Work out the finished part from the listing and answer in its coordinate system (mm). A direction names the side the tool comes from. Round coordinates to 2 decimals unless told otherwise and drop trailing zeros. Order: outer loops, then holes, each group sorted by start corner. A loop starts at its lowest first (then second) coordinate and runs counter-clockwise, first axis right, second up. Notation, with made-up numbers: (54.25, 12.25) - (105.25, 12.25) arc R28 ccw to (105.25, 39.25) - close; hole circle Ø9 at (74.25, -3.5). An arc over 180 degrees is marked (long way). Put each result on its own line as item: value.
```python
from build123d import *

# Parameters (mm, degrees)
SKETCH_1_W          = 55
SKETCH_1_H          = 100
EXTRUDE_1_DEPTH     = 30
CUT_EXTRUDE_1_DEPTH = 81.156097709
SKETCH_3_W          = 50
SKETCH_3_H          = 95
CUT_EXTRUDE_2_DEPTH = 25
FILLET_1_R          = 5
SKETCH_5_R          = 3
EXTRUDE_2_DEPTH     = 25
SKETCH_6_W          = 15
SKETCH_6_H          = 23
CUT_EXTRUDE_4_DEPTH = 5
CHAMFER_1_SIZE      = 4
SKETCH_7_R          = 5
EXTRUDE_3_DEPTH     = 5
SKETCH_8_R          = 2.75
CUT_EXTRUDE_5_DEPTH = 5


with BuildPart() as part:
    # 草圖1 → 填料-伸長1 (new body)
    with BuildSketch(Plane.XY):
        Rectangle(SKETCH_1_W, SKETCH_1_H)
    extrude(amount=EXTRUDE_1_DEPTH)

    # 草圖2 → 除料-伸長1 (cut, through all)
    with BuildSketch(Plane.ZY.offset(27.5)):
        with BuildLine():
            Line((13, 39.5), (30, 39.5))
            Line((30, 39.5), (30, 30.5))
            Line((30, 30.5), (13, 30.5))
            ThreePointArc((13, 30.5), (8.5, 35), (13, 39.5))
        make_face()
    extrude(amount=-CUT_EXTRUDE_1_DEPTH, mode=Mode.SUBTRACT)

    # 草圖3 → 除料-伸長2 (cut)
    with BuildSketch(Plane.XY.offset(30)):
        Rectangle(SKETCH_3_W, SKETCH_3_H)
    extrude(amount=-CUT_EXTRUDE_2_DEPTH, mode=Mode.SUBTRACT)

    # 圓角1
    fillet_1_edges = [part.edges().sort_by_distance(p)[0] for p in [
        (25, 47.5, 17.5),
        (-25, -47.5, 17.5),
        (25, -47.5, 17.5),
        (-25, 47.5, 17.5),
        (27.5, -50, 15),
        (-27.5, -50, 15),
        (-27.5, 50, 15),
        (27.5, 50, 15),
    ]]
    fillet(fillet_1_edges, radius=FILLET_1_R)

    # 草圖5 → 填料-伸長2 (add)
    with BuildSketch(Plane.XY.offset(5)):
        with Locations(Location((11, -35, 0), (0, 0, 180))):
            Circle(SKETCH_5_R)
    extrude(amount=EXTRUDE_2_DEPTH)

    # 草圖6 → 除料-伸長4 (cut)
    with BuildSketch(Plane.XZ.offset(50)):
        with Locations((0, 18.5)):
            Rectangle(SKETCH_6_W, SKETCH_6_H)
    extrude(amount=-CUT_EXTRUDE_4_DEPTH, mode=Mode.SUBTRACT)

    # 導角1
    # the kernel refuses this chamfer: 4 mm, written as the material it adds along each edge
    with BuildSketch(Plane(origin=(-20, -42.5, 5), x_dir=(-1, 0, 0), z_dir=(0, 1, 0))) as chamfer_1_piece_1:
        Polygon((5, CHAMFER_1_SIZE), (5 - CHAMFER_1_SIZE, 0), (5, 0), align=None)
    revolve(axis=Axis((-20, -42.5, 5), (0, 0, 1)), revolution_arc=90)
    with BuildSketch(Plane(origin=(-25, 42.5, 5), x_dir=(-0.027495876610586487, 0, 0.9996219169112968), z_dir=(0, -1, 0))) as chamfer_1_piece_2_section:
        Polygon((CHAMFER_1_SIZE * 0.999621916911, -CHAMFER_1_SIZE * 0.0274958766106), (-CHAMFER_1_SIZE * 0.0274958766106, -CHAMFER_1_SIZE * 0.999621916911), (0, 0), align=None)
    chamfer_1_piece_2 = extrude(amount=85, mode=Mode.PRIVATE)
    chamfer_1_piece_2 = chamfer_1_piece_2 - Plane(origin=(-23.679821879, 35, 13), x_dir=(0, -1, 0), z_dir=(-1, 0, 0)) * Cylinder(4.5, 186, mode=Mode.PRIVATE)
    add(chamfer_1_piece_2)
    with BuildSketch(Plane(origin=(-20, 42.5, 5), x_dir=(-1, 0, 0), z_dir=(0, -1, 0))) as chamfer_1_piece_3:
        Polygon((5 - CHAMFER_1_SIZE, 0), (5, -CHAMFER_1_SIZE), (5, 0), align=None)
    revolve(axis=Axis((-20, 42.5, 5), (0, 0, -1)), revolution_arc=90)
    with BuildSketch(Plane(origin=(20, 47.5, 5), x_dir=(0, -0.9996219169112968, -0.027495876610586296), z_dir=(-1, 0, 0))) as chamfer_1_piece_4:
        Polygon((CHAMFER_1_SIZE * 0.999621916911, CHAMFER_1_SIZE * 0.0274958766106), (-CHAMFER_1_SIZE * 0.0274958766106, CHAMFER_1_SIZE * 0.999621916911), (0, 0), align=None)
    extrude(amount=40)
    with BuildSketch(Plane(origin=(20, 42.5, 5), x_dir=(1, 0, 0), z_dir=(0, -1, 0))) as chamfer_1_piece_5:
        Polygon((5 - CHAMFER_1_SIZE, 0), (5, CHAMFER_1_SIZE), (5, 0), align=None)
    revolve(axis=Axis((20, 42.5, 5), (0, 0, 1)), revolution_arc=90)
    with BuildSketch(Plane(origin=(25, -42.5, 5), x_dir=(0.027495876610586487, 0, 0.9996219169112968), z_dir=(0, 1, 0))) as chamfer_1_piece_6_section:
        Polygon((CHAMFER_1_SIZE * 0.999621916911, -CHAMFER_1_SIZE * 0.0274958766106), (-CHAMFER_1_SIZE * 0.0274958766106, -CHAMFER_1_SIZE * 0.999621916911), (0, 0), align=None)
    chamfer_1_piece_6 = extrude(amount=85, mode=Mode.PRIVATE)
    chamfer_1_piece_6 = chamfer_1_piece_6 - Plane(origin=(23.679821879, 35, 13), x_dir=(0, -1, 0), z_dir=(-1, 0, 0)) * Cylinder(4.5, 186, mode=Mode.PRIVATE)
    add(chamfer_1_piece_6)
    with BuildSketch(Plane(origin=(20, -42.5, 5), x_dir=(0, -1, 0), z_dir=(-1, 0, 0))) as chamfer_1_piece_7:
        Polygon((5, CHAMFER_1_SIZE), (5 - CHAMFER_1_SIZE, 0), (5, 0), align=None)
    revolve(axis=Axis((20, -42.5, 5), (0, 0, 1)), revolution_arc=90)
    with BuildSketch(Plane(origin=(-20, -47.5, 5), x_dir=(0, -0.027495876610585623, 0.9996219169112968), z_dir=(1, 0, 0))) as chamfer_1_piece_8_section:
        Polygon((CHAMFER_1_SIZE * 0.999621916911, -CHAMFER_1_SIZE * 0.0274958766106), (-CHAMFER_1_SIZE * 0.0274958766106, -CHAMFER_1_SIZE * 0.999621916911), (0, 0), align=None)
    chamfer_1_piece_8 = extrude(amount=40, mode=Mode.PRIVATE)
    chamfer_1_piece_8 = split(chamfer_1_piece_8, bisect_by=Plane(origin=(-13.75, -46.917717373, 7), z_dir=(0, 0, 1)), keep=Keep.TOP, mode=Mode.PRIVATE)
    chamfer_1_piece_8 = split(chamfer_1_piece_8, bisect_by=Plane(origin=(-7.5, -46.917717373, 7.727438446), z_dir=(-1, 0, 0)), keep=Keep.TOP, mode=Mode.PRIVATE)
    add(chamfer_1_piece_8)
    with BuildSketch(Plane(origin=(-20, -47.5, 5), x_dir=(0, -0.027495876610585623, 0.9996219169112968), z_dir=(1, 0, 0))) as chamfer_1_piece_9_section:
        Polygon((CHAMFER_1_SIZE * 0.999621916911, -CHAMFER_1_SIZE * 0.0274958766106), (-CHAMFER_1_SIZE * 0.0274958766106, -CHAMFER_1_SIZE * 0.999621916911), (0, 0), align=None)
    chamfer_1_piece_9 = extrude(amount=40, mode=Mode.PRIVATE)
    chamfer_1_piece_9 = split(chamfer_1_piece_9, bisect_by=Plane(origin=(-13.75, -45.926395663, 7), z_dir=(0, 0, -1)), keep=Keep.TOP, mode=Mode.PRIVATE)
    chamfer_1_piece_9 = split(chamfer_1_piece_9, bisect_by=Plane(origin=(-7.5, -45.926395663, 5.832937159), z_dir=(-1, 0, 0)), keep=Keep.TOP, mode=Mode.PRIVATE)
    add(chamfer_1_piece_9)
    with BuildSketch(Plane(origin=(-20, -47.5, 5), x_dir=(0, -0.027495876610585623, 0.9996219169112968), z_dir=(1, 0, 0))) as chamfer_1_piece_10_section:
        Polygon((CHAMFER_1_SIZE * 0.999621916911, -CHAMFER_1_SIZE * 0.0274958766106), (-CHAMFER_1_SIZE * 0.0274958766106, -CHAMFER_1_SIZE * 0.999621916911), (0, 0), align=None)
    chamfer_1_piece_10 = extrude(amount=40, mode=Mode.PRIVATE)
    chamfer_1_piece_10 = split(chamfer_1_piece_10, bisect_by=Plane(origin=(7.5, -45.926395663, 5.832937159), z_dir=(-1, 0, 0)), keep=Keep.TOP, mode=Mode.PRIVATE)
    chamfer_1_piece_10 = split(chamfer_1_piece_10, bisect_by=Plane(origin=(0, -45.926395663, 7), z_dir=(0, 0, -1)), keep=Keep.TOP, mode=Mode.PRIVATE)
    chamfer_1_piece_10 = split(chamfer_1_piece_10, bisect_by=Plane(origin=(-7.5, -45.926395663, 5.832937159), z_dir=(1, 0, 0)), keep=Keep.TOP, mode=Mode.PRIVATE)
    add(chamfer_1_piece_10)
    with BuildSketch(Plane(origin=(-20, -47.5, 5), x_dir=(0, -0.027495876610585623, 0.9996219169112968), z_dir=(1, 0, 0))) as chamfer_1_piece_11_section:
        Polygon((CHAMFER_1_SIZE * 0.999621916911, -CHAMFER_1_SIZE * 0.0274958766106), (-CHAMFER_1_SIZE * 0.0274958766106, -CHAMFER_1_SIZE * 0.999621916911), (0, 0), align=None)
    chamfer_1_piece_11 = extrude(amount=40, mode=Mode.PRIVATE)
    chamfer_1_piece_11 = split(chamfer_1_piece_11, bisect_by=Plane(origin=(7.5, -46.917717373, 7.727438446), z_dir=(1, 0, 0)), keep=Keep.TOP, mode=Mode.PRIVATE)
    chamfer_1_piece_11 = split(chamfer_1_piece_11, bisect_by=Plane(origin=(13.75, -46.917717373, 7), z_dir=(0, 0, 1)), keep=Keep.TOP, mode=Mode.PRIVATE)
    add(chamfer_1_piece_11)
    with BuildSketch(Plane(origin=(-20, -47.5, 5), x_dir=(0, -0.027495876610585623, 0.9996219169112968), z_dir=(1, 0, 0))) as chamfer_1_piece_12_section:
        Polygon((CHAMFER_1_SIZE * 0.999621916911, -CHAMFER_1_SIZE * 0.0274958766106), (-CHAMFER_1_SIZE * 0.0274958766106, -CHAMFER_1_SIZE * 0.999621916911), (0, 0), align=None)
    chamfer_1_piece_12 = extrude(amount=40, mode=Mode.PRIVATE)
    chamfer_1_piece_12 = split(chamfer_1_piece_12, bisect_by=Plane(origin=(7.5, -45.926395663, 5.832937159), z_dir=(1, 0, 0)), keep=Keep.TOP, mode=Mode.PRIVATE)
    chamfer_1_piece_12 = split(chamfer_1_piece_12, bisect_by=Plane(origin=(13.75, -45.926395663, 7), z_dir=(0, 0, -1)), keep=Keep.TOP, mode=Mode.PRIVATE)
    add(chamfer_1_piece_12)
    # the kernel refuses this chamfer: 4 mm, written as the material it takes off along each edge
    with BuildSketch(Plane(origin=(-27.5, 45, 0), x_dir=(-0.027495876610586494, 0, 0.9996219169112968), z_dir=(0, -1, 0)), Plane(origin=(27.5, -45, 0), x_dir=(0.027495876610586494, 0, 0.9996219169112968), z_dir=(0, 1, 0))) as chamfer_1_2_piece_1:
        Polygon((CHAMFER_1_SIZE * 0.999621916911, -CHAMFER_1_SIZE * 0.0274958766106), (-CHAMFER_1_SIZE * 0.0274958766106, -CHAMFER_1_SIZE * 0.999621916911), (0, 0), align=None)
    extrude(amount=90, mode=Mode.SUBTRACT)
    with BuildSketch(Plane(origin=(-22.5, -45, 0), x_dir=(0, -1, 0), z_dir=(1, 0, 0))) as chamfer_1_2_piece_2:
        Polygon((5, -CHAMFER_1_SIZE), (5 - CHAMFER_1_SIZE, 0), (5, 0), align=None)
    revolve(axis=Axis((-22.5, -45, 0), (0, 0, -1)), revolution_arc=90, mode=Mode.SUBTRACT)
    with BuildSketch(Plane(origin=(-22.5, 45, 0), x_dir=(-1, 0, 0), z_dir=(0, -1, 0))) as chamfer_1_2_piece_3:
        Polygon((5, -CHAMFER_1_SIZE), (5 - CHAMFER_1_SIZE, 0), (5, 0), align=None)
    revolve(axis=Axis((-22.5, 45, 0), (0, 0, -1)), revolution_arc=90, mode=Mode.SUBTRACT)
    with BuildSketch(Plane(origin=(-22.5, -50, 0), x_dir=(0, -0.02749587661058563, 0.9996219169112968), z_dir=(1, 0, 0)), Plane(origin=(22.5, 50, 0), x_dir=(0, 0.02749587661058563, 0.9996219169112968), z_dir=(-1, 0, 0))) as chamfer_1_2_piece_4:
        Polygon((CHAMFER_1_SIZE * 0.999621916911, -CHAMFER_1_SIZE * 0.0274958766106), (-CHAMFER_1_SIZE * 0.0274958766106, -CHAMFER_1_SIZE * 0.999621916911), (0, 0), align=None)
    extrude(amount=45, mode=Mode.SUBTRACT)
    with BuildSketch(Plane(origin=(22.5, -45, 0), x_dir=(0, -1, 0), z_dir=(-1, 0, 0))) as chamfer_1_2_piece_5:
        Polygon((5, CHAMFER_1_SIZE), (5 - CHAMFER_1_SIZE, 0), (5, 0), align=None)
    revolve(axis=Axis((22.5, -45, 0), (0, 0, 1)), revolution_arc=90, mode=Mode.SUBTRACT)
    with BuildSketch(Plane(origin=(22.5, 45, 0), x_dir=(1, 0, 0), z_dir=(0, -1, 0))) as chamfer_1_2_piece_6:
        Polygon((5, CHAMFER_1_SIZE), (5 - CHAMFER_1_SIZE, 0), (5, 0), align=None)
    revolve(axis=Axis((22.5, 45, 0), (0, 0, 1)), revolution_arc=90, mode=Mode.SUBTRACT)

    # 草圖7 → 填料-伸長3 (add)
    with BuildSketch(Plane.XY.offset(5)):
        with Locations(Location((11, -35, 0), (0, 0, 180))):
            Circle(SKETCH_7_R)
    extrude(amount=EXTRUDE_3_DEPTH)

    # 草圖8 → 除料-伸長5 (cut)
    with BuildSketch(Plane.XZ.offset(50)):
        with Locations(Location((-12, 18, 0), (0, 0, 270))):
            Circle(SKETCH_8_R)
    extrude(amount=-CUT_EXTRUDE_5_DEPTH, mode=Mode.SUBTRACT)


solid = part.part
```
1) Given pin 1 Ø3 at (x, z) = (-26.5, 23.5) entering from +Y; pin 2 Ø3 at (x, z) = (-27, 24.5) entering from -Y; pin 3 Ø5 at (x, z) = (-12, 18) entering from -Y; pin 4 Ø1.6 at (y, z) = (38.5, 18) entering from -X, each flat-ended and moving along its own axis, determine where each tip first touches the part or whether it passes through.
Findings below:
pin 1: stops at y = 49.33
pin 2: stops at y = -49
pin 3: stops at y = 47.5
pin 4: passes through
2) A cutting plane is placed at D-D on z = 2.5. Write down the section's boundary in (x, y).
Findings below:
outline: (-26, -45) arc R3.5 ccw to (-22.5, -48.5) - (22.5, -48.5) arc R3.5 ccw to (26, -45) - (26, 45) arc R3.5 ccw to (22.5, 48.5) - (-22.5, 48.5) arc R3.5 ccw to (-26, 45) - close
3) A cutting plane is placed at C-C on y = -31. Write down the section's boundary in (x, z).
Findings below:
outline: (-27.5, 4) - (-23.5, 0) - (23.5, 0) - (27.5, 4) - (27.5, 30) - (25, 30) - (25, 9) - (21, 5) - (14, 5) - (14, 10) - (8, 10) - (8, 5) - (-21, 5) - (-25, 9) - (-25, 30) - (-27.5, 30) - close
4) For faces 1 (the cylindrical face through (23.57, 46, 19.35)), 2 (the flat face through (-25.5, 0.6, 2)), 3 (the flat face through (-26, 30.5, 22)), 4 (the cylindrical face through (-10.141, -48.768, 20.027)), determine the directions among +Z, -Z, +X, -X, +Y, -Y from which every point of the face is accessible in a straight line to the end or side of a thin tool.
Findings below:
face 1: +Z
face 2: -Z, -X, +Y, -Y
face 3: +Z, +X, -X
face 4: -Y
5) A cutting plane is placed at A-A on z = 27. Give the number of separate pieces and of enclosed holes in the cut face, then the cut area to 3 significant figures.
Findings below:
separate pieces: 4
enclosed holes: 0
area: 696 mm2
6) For a pull along X with two mould halves and no side action, classify faces 5 (the conical face through (-24.58, -47.12, 1.97)), 6 (the flat face through (-7.5, -49, 19)), 7 (the conical face through (24.62, 47.08, 1.97)) as pulls with the +X half, pulls with the -X half, needs draft (parallel to the pull), parting line crosses it, or undercut.
Findings below:
face 5: pulls with the -X half
face 6: undercut
face 7: pulls with the +X half
7) Straight lines are drawn through the part: L1, parallel to X at y = -35, z = 11; L2, parallel to X at y = 20, z = 25.5; L3, parallel to Y at x = 17.5, z = 15.5. For each, find the intervals that lie inside material, in ascending order. Write a range as from..to.
Findings below:
L1: x = -27.5..-25, 8..14, 25..27.5
L2: x = -27.5..-25, 25..27.5
L3: y = -50..-47.5, 47.5..50
8) A cutting plane is placed at B-B on x = -12. Write down the section's boundary in (y, z), then the cut area to 3 significant figures.
Findings below:
outline: (-50, 4) - (-46, 0) - (46, 0) - (50, 4) - (50, 30) - (47.5, 30) - (47.5, 9) - (43.5, 5) - (-43.5, 5) - (-47.5, 9) - (-47.5, 15.25) - (-50, 15.25) - close; (-50, 20.75) - (-47.5, 20.75) - (-47.5, 30) - (-50, 30) - close
area: 611 mm2
